Geometry: see drawing. Coordinates: mm, zero at the bounding-box minimum. A direction names the side the tool comes from. Coordinates: 2 decimals unless noted, no trailing zeros. Loops run counter-clockwise (first coordinate to the right, second up) from the corner with the lowest first, then second, coordinate; pieces in that order, holes last. Notation, with made-up numbers: (87.5, 27) - (110.5, 27) arc R26 ccw to (110.5, 64) - close; hole circle Ø5 at (-19.75, -19.75). An arc over 180 degrees is marked (long way). Answer in a Markdown table with one row per item.
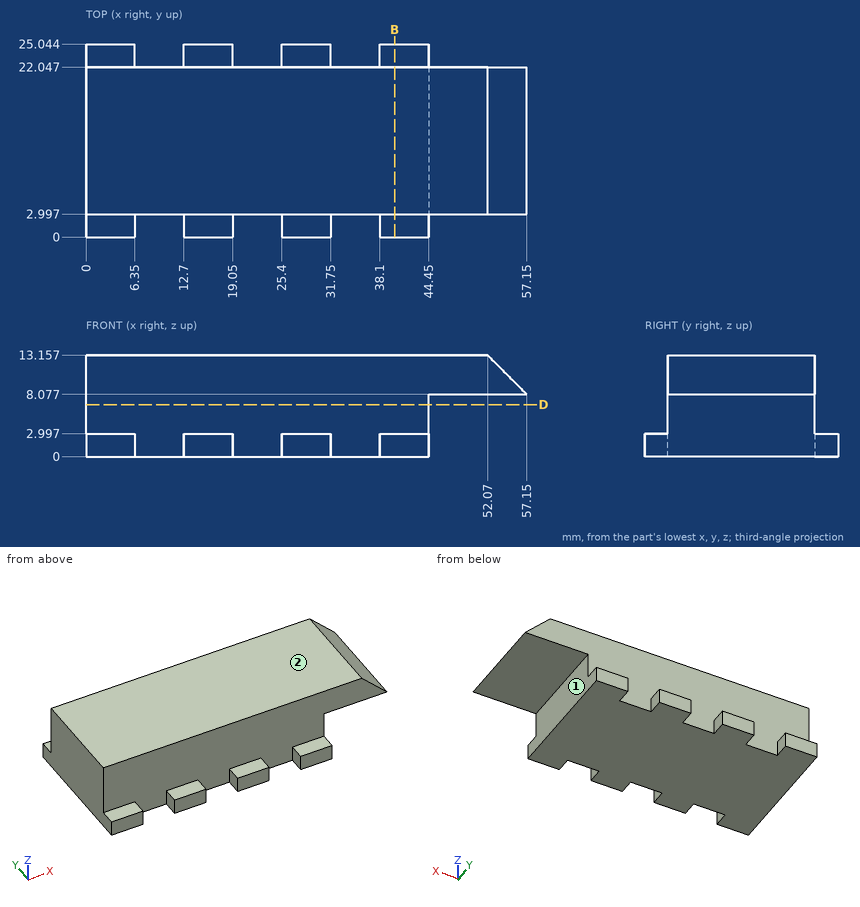
(1) Access query for the marked faces 1 and 2. Directions: +Z, -Z, +X, -X, +Y, -Y. A direction counts if a zero-diameter tool reaches every point of the face in a straight line with its end or side. Return the directions, or none.
Verdict:
| item | result |
|---|---|
| face 1 | -Z, +X, +Y, -Y |
| face 2 | +Z, +X, -X, +Y, -Y |
(2) Cut plane B-B on x = 40. Output: boundary loops of the cut face in (y, z) (1 decimal).
Verdict:
| item | result |
|---|---|
| outline | (0, 0) - (25, 0) - (25, 3) - (22, 3) - (22, 13.2) - (3, 13.2) - (3, 3) - (0, 3) - close |
(3) Cut plane D-D on z = 6.75. Output: boundary loops of the cut face in (x, y), then the cut area to 3 significant figures.
Verdict:
| item | result |
|---|---|
| outline | (0, 3) - (44.45, 3) - (44.45, 22.05) - (0, 22.05) - close |
| area | 847 mm² |
(4) First-contact query: pin 1 Ø4 at (x, z) = (21.5, 9) entering from -Y; pin 2 Ø3.5 at (y, z) = (2, 1.5) entering from +X; pin 3 Ø1.5 at (x, y) = (2.5, 23.5) entering from +Z. Flat tips, straight axial feed; report the tip coordinate or a pass-through.
Verdict:
| item | result |
|---|---|
| pin 1 | stops at y = 3 |
| pin 2 | stops at x = 44.45 |
| pin 3 | stops at z = 3 |
(5) Ray query, probe 1 along Y at (x, z) = (25, 5.5); probe 2 along X at (y, z) = (10, 4); probe 3 along Z at (x, y) = (17, 23.5). Return the intervals inside material, ascending.
Verdict:
| item | result |
|---|---|
| probe 1 | y = 3 to 22.05 |
| probe 2 | x = 0 to 44.45 |
| probe 3 | z = 0 to 3 |
